```python
from build123d import *

# Parameters (mm, degrees)
F0_W     = 57.15
F0_H     = 95.25
F1_DEPTH = 63.5
F2_R     = 12.7
F2_R_2   = 25.4
F3_DEPTH = 25.4
F4_SIZE  = 6.35


with BuildPart() as f1:
    # F0 (on Front) → F1 (new body)
    with BuildSketch(Plane.XZ):
        Rectangle(F0_W, F0_H)
    extrude(amount=F1_DEPTH)

    # F2 (on face) → F3 (cut)
    with BuildSketch(Plane(origin=(0, 0, 0), x_dir=(-1, 0, 0), z_dir=(0, 1, 0))):
        with Locations((0, 28.575)):
            Circle(F2_R)
        with Locations((0, -15.875)):
            Circle(F2_R_2)
    extrude(amount=-F3_DEPTH, mode=Mode.SUBTRACT)

    # F4
    f4_edges = [f1.edges().sort_by_distance(p)[0] for p in [
        (-28.575, -31.75, 47.625),
        (28.575, -31.75, 47.625),
        (28.575, -31.75, -47.625),
        (-28.575, -31.75, -47.625),
    ]]
    chamfer(f4_edges, length=F4_SIZE)


solid = f1.part
```
Could you check a few things on this model? Use its own coordinates, in mm. A direction names the side the tool comes from. Coordinates: 2 decimals unless noted, no trailing zeros. Write each loop counter-clockwise with the first axis right and the second up, starting at its lowest first coordinate (ties: lowest second). Pieces come first, ordered by that corner, then holes. Notation, with made-up numbers: M 64,84.5 L 90,84.5 A24 ccw 90,107.5 Z; hole C 62.25,59 d3. An arc over 180 degrees is marked long. Answer as CSV lines item,"result". Start each with the question number.
1) For faces 1 (the flat face through (0, -63.5, 1)), 2 (the cylindrical face through (2.753, -12.522, 16.177)), which set-ups out of +Z, -Z, +X, -X, +Y, -Y let a thin tool reach every point of the face, with its end or its side?
2) I want a section at B-B, the plane y = -8.5. Please give me the cut outline in (x, z) (3 decimals).
3) Please list where these lines run through material, in increasing order: line 1 (Z direction, x = 0, y = -20) (3 decimals); line 2 (Y direction, x = 5, z = 30.5); line 3 (X direction, y = -20, z = 25.5) (3 decimals). Write a range as from..to.
4) I want a section at A-A, the plane x = 0. Please give me the cut outline in (y, z) (3 decimals), and give its area (3 significant figures).
5) I want a section at C-C, the plane z = 19.5. Please give me the cut outline in (x, y) (1 decimal), and give its area (3 significant figures).
6) We'd pull the mould along Z, two halves only. Please class faces 3 (the cylindrical face through (20.157, -12.522, -31.331)), 4 (the flat face through (0, 0, 11)), 5 (the flat face through (-25.36, -31.31, -44.49)): +Z half, -Z half, draft (parallel to the pull), parting line (faces both ways), or undercut.
7) For P1, Ø10, axis at x = -0.5, z = -11.5, coming from the +Y side, with a flat end and sliding along its axis, tell me the tip position at first contact or that it passes through.
8) I want a section at D-D, the plane x = 23.5. Please give me the cut outline in (y, z).
Data:
1,face 1,"+Z, -Z, +X, -X, -Y"
1,face 2,"+Y"
2,outline,"M -28.575,-41.275 L -22.225,-47.625 L 22.225,-47.625 L 28.575,-41.275 L 28.575,41.275 L 22.225,47.625 L -22.225,47.625 L -28.575,41.275 Z; hole C 0,-15.875 d50.8; hole C 0,28.575 d25.4"
3,line 1,"z = -47.625..-41.275, 9.525..15.875, 41.275..47.625"
3,line 2,"y = -63.5..-25.4"
3,line 3,"x = -28.575..-12.322, 12.322..28.575"
4,outline,"M -63.5,-47.625 L 0,-47.625 L 0,-41.275 L -25.4,-41.275 L -25.4,9.525 L 0,9.525 L 0,15.875 L -25.4,15.875 L -25.4,41.275 L 0,41.275 L 0,47.625 L -63.5,47.625 Z"
4,area,"4,110 mm^2"
5,outline,"M -28.6,-63.5 L 28.6,-63.5 L 28.6,0 L 8.9,0 L 8.9,-25.4 L -8.9,-25.4 L -8.9,0 L -28.6,0 Z"
5,area,"3,180 mm^2"
6,face 3,"undercut"
6,face 4,"draft"
6,face 5,"-Z half"
7,P1,"stops at y = -25.4"
8,outline,"M -63.5,-46.35 L 0,-46.35 L 0,-25.51 L -25.4,-25.51 L -25.4,-6.24 L 0,-6.24 L 0,46.35 L -63.5,46.35 Z"
